Input: dimensioned drawing with shaded views. Units: mm. Origin: part minimum x, y, z. Coordinates: 2 decimals unless noted, no trailing zeros. Order: outer loops, then holes, each group sorted by start corner. A loop starts at its lowest first (then second) coordinate and runs counter-clockwise, first axis right, second up. Notation, with made-up numbers: M 77,71 L 100,71 A20 cw 100,94 Z; hole C -1.5,35 d2. An arc over 180 degrees is marked long. Use CSV: the item, a comma, the result in double quotes. Start each with the question number.
1. Section query C-C on x = 135. Return the cut outline in (y, z).
2. Section query B-B on y = 2.1. Return the cut outline in (x, z).
3. First-contact query: P1, Ø3, axis at x = 149.68, z = 215.75, coming from the -Y side. Flat tip, straight axial feed; report the tip coordinate or a pass-through.
4. Section query A-A on z = 201.5. Return the cut outline in (x, y).
5. Material intervals for line 1 (X direction, y = 2.1, z = 201.5); line 2 (X direction, y = 0.9, z = 215.75); line 3 (X direction, y = 1.8, z = 186) (1 decimal), sorted ascending.
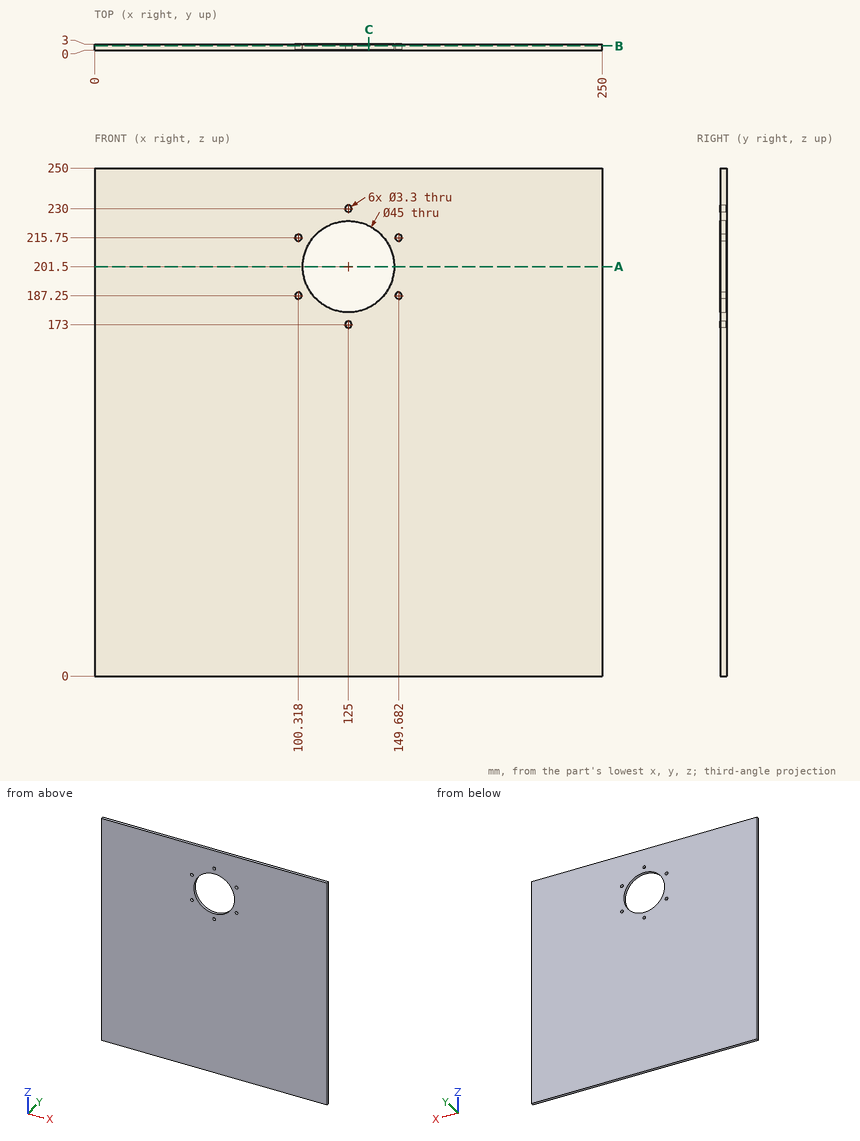
Results list:
1,outline,"M 0,0 L 3,0 L 3,181.34 L 0,181.34 Z; M 0,221.66 L 3,221.66 L 3,250 L 0,250 Z"
2,outline,"M 0,0 L 250,0 L 250,250 L 0,250 Z; hole C 100.32,187.25 d3.3; hole C 100.32,215.75 d3.3; hole C 125,201.5 d45; hole C 125,173 d3.3; hole C 125,230 d3.3; hole C 149.68,187.25 d3.3; hole C 149.68,215.75 d3.3"
3,P1,"passes through"
4,outline,"M 0,0 L 102.5,0 L 102.5,3 L 0,3 Z; M 147.5,0 L 250,0 L 250,3 L 147.5,3 Z"
5,line 1,"x = 0 to 102.5, 147.5 to 250"
5,line 2,"x = 0 to 98.67, 101.97 to 107.59, 142.41 to 148.03, 151.33 to 250"
5,line 3,"x = 0 to 99.2, 101.4 to 108.7, 141.3 to 148.6, 150.8 to 250"
